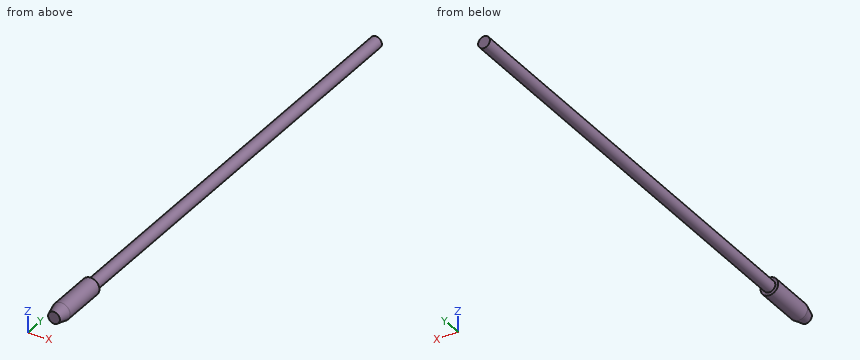
```python
from build123d import *

# Parameters (mm, degrees)
SKETCH19_R          = 5
BOSS_EXTRUDE1_DEPTH = 390
SKETCH25_R          = 7.5
BOSS_EXTRUDE2_DEPTH = 40
SKETCH26_R          = 7.5
SKETCH27_R          = 5


with BuildPart() as part:
    # Sketch19 → Boss-Extrude1 (new body)
    with BuildSketch(Plane(origin=(0, 0, 0), x_dir=(1, 0, 0), z_dir=(0, 1, 0))):
        with Locations(Location((276.355570331, 125.849309684, 0), (0, 0, 270))):
            Circle(SKETCH19_R)
    extrude(amount=-BOSS_EXTRUDE1_DEPTH)

    # Sketch25 → Boss-Extrude2 (add)
    with BuildSketch(Plane.XZ.offset(390)):
        with Locations(Location((276.355570331, -125.849309684, 0), (0, 0, 270))):
            Circle(SKETCH25_R)
    extrude(amount=BOSS_EXTRUDE2_DEPTH)

    # Sketch26 → Loft1 section 0
    with BuildSketch(Plane.XZ.offset(430)):
        with Locations((276.355570331, -125.849309684)):
            Circle(SKETCH26_R)
    # Sketch27 → Loft1 section 1
    with BuildSketch(Plane(origin=(0, -440, 0), x_dir=(-1, 0, 0), z_dir=(0, -1, 0))):
        with Locations((-276.355570331, 125.849309684)):
            Circle(SKETCH27_R)
    loft()


solid = part.part
```
Here's how the part is built. I have some questions about the finished solid (model axes, mm). Give positions to 0.01 mm unless a question says otherwise; leave off trailing zeros. Order: outer loops, then holes, each group sorted by start corner. A loop starts at its lowest first (then second) coordinate and runs counter-clockwise, first axis right, second up. Notation, with made-up numbers: (85.5, 11.25) -> (104.5, 11.25) arc R19 ccw to (104.5, 28.25) -> close; hole circle Ø2 at (0, 52). An arc over 180 degrees is marked (long way). Use CSV: the item, a comma, the result in double quotes. Start each with the question number.
Item 1: Suppose I cut it at A-A (y = -223). List the corners of the cut face in (x, z) for me, and give its area (3 significant figures).
Item 2: If I drill on probe 1 along Z at (x, y) = (276.75, -83); probe 2 along X at (y, z) = (-400, -126.75); probe 3 along X at (y, z) = (-362.5, -125.25), over which ranges is the centre line in solid material (lowest first)? Write a range as [from, to].
Item 3: I'm going to push flat-ended pins straight in: P1, Ø5, axis at x = 282, y = -55.5, coming from the -Z side; P2, Ø1.5, axis at y = -288, z = -121.5, coming from the +X side; P3, Ø4, axis at y = -186, z = -128, coming from the +X side. Where does each tip first touch, or does it pass through?
Answer block:
1,outline,"circle Ø10 at (276.36, -125.85)"
1,area,"78.5 mm^2"
2,probe 1,"z = [-130.83, -120.86]"
2,probe 2,"x = [268.91, 283.8]"
2,probe 3,"x = [271.39, 281.32]"
3,P1,"stops at z = -129.74"
3,P2,"stops at x = 279.83"
3,P3,"stops at x = 281.35"
